```python
from build123d import *

# Parameters (mm, degrees)
EXTRUDE_1_DEPTH     = 2
SKETCH_2_R          = 1.05
CUT_EXTRUDE_1_DEPTH = 2
SKETCH_3_R          = 1.05
CUT_EXTRUDE_2_DEPTH = 2
FILLET_1_R          = 5
FILLET_2_R          = 1.5
SKETCH_5_R          = 1.6
CUT_EXTRUDE_4_DEPTH = 10
SKETCH_6_R          = 1.6
CUT_EXTRUDE_5_DEPTH = 10
CUT_EXTRUDE_6_DEPTH = 10
FILLET_3_R          = 2
FILLET_4_R          = 1.5
SKETCH_10_R         = 1.05
CUT_EXTRUDE_7_DEPTH = 10


with BuildPart() as part:
    # 草图1 → 凸台-拉伸1 (new body)
    with BuildSketch(Plane.XY):
        with BuildLine():
            Line((-53.112698372, 0), (-53.112698372, 20))
            Line((-53.112698372, 20), (-60.112698372, 20))
            Line((-60.112698372, 20), (-60.112698372, -60.112698372))
            Line((-60.112698372, -60.112698372), (10, -60.112698372))
            Line((10, -60.112698372), (10, -53.112698372))
            Line((10, -53.112698372), (0, -53.112698372))
            ThreePointArc((0, -53.112698372), (-37.556349186, -37.556349186), (-53.112698372, 0))
        make_face()
    extrude(amount=EXTRUDE_1_DEPTH)

    # 草图2 → 切除-拉伸1 (cut)
    with BuildSketch(Plane.XY.offset(2)):
        with Locations((5, -55.112698372)):
            Circle(SKETCH_2_R)
    extrude(amount=-CUT_EXTRUDE_1_DEPTH, mode=Mode.SUBTRACT)

    # 草图3 → 切除-拉伸2 (cut)
    with BuildSketch(Plane.XY.offset(2)):
        with Locations((-0.799997093, -55.106891824)):
            Circle(SKETCH_3_R)
        with Locations((-6.964981152, -54.670819999)):
            Circle(SKETCH_3_R)
        with Locations((-13.042376532, -53.547230893)):
            Circle(SKETCH_3_R)
        with Locations((-18.95575646, -51.750254288)):
            Circle(SKETCH_3_R)
        with Locations((-24.630756751, -49.30248821)):
            Circle(SKETCH_3_R)
        with Locations((-29.996010986, -46.234714737)):
            Circle(SKETCH_3_R)
        with Locations((-34.984047978, -42.5855129)):
            Circle(SKETCH_3_R)
        with Locations((-39.532140269, -38.400773529)):
            Circle(SKETCH_3_R)
        with Locations((-43.583092958, -33.733122151)):
            Circle(SKETCH_3_R)
        with Locations((-47.085962967, -28.641257189)):
            Circle(SKETCH_3_R)
        with Locations((-49.996699671, -23.1892118)):
            Circle(SKETCH_3_R)
        with Locations((-52.278698867, -17.445548618)):
            Circle(SKETCH_3_R)
        with Locations((-53.903263093, -11.48249754)):
            Circle(SKETCH_3_R)
        with Locations((-54.84996251, -5.375047393)):
            Circle(SKETCH_3_R)
        with Locations((-55.106891824, 0.799997093)):
            Circle(SKETCH_3_R)
    extrude(amount=-CUT_EXTRUDE_2_DEPTH, mode=Mode.SUBTRACT)

    # 圆角1
    fillet_1_edges = [part.edges().sort_by_distance(p)[0] for p in [
        (-60.112698372, -60.112698372, 1),
    ]]
    fillet(fillet_1_edges, radius=FILLET_1_R)

    # 圆角2
    fillet_2_edges = [part.edges().sort_by_distance(p)[0] for p in [
        (-60.112698372, 20, 1),
        (-53.112698372, 20, 1),
        (10, -53.112698372, 1),
        (10, -60.112698372, 1),
    ]]
    fillet(fillet_2_edges, radius=FILLET_2_R)

    # 草图5 → 切除-拉伸4 (cut)
    with BuildSketch(Plane.XY.offset(2)):
        with Locations((-57.199529996, -26.67257888)):
            Circle(SKETCH_5_R)
    extrude(amount=-CUT_EXTRUDE_4_DEPTH, mode=Mode.SUBTRACT)

    # 草图6 → 切除-拉伸5 (cut)
    with BuildSketch(Plane(origin=(0, 0, 0), x_dir=(-1, 0, 0), z_dir=(0, 0, -1))):
        with Locations((27, -57.112698372)):
            Circle(SKETCH_6_R)
        with Locations((47, -57.112698372)):
            Circle(SKETCH_6_R)
    extrude(amount=-CUT_EXTRUDE_5_DEPTH, mode=Mode.SUBTRACT)

    # 草图7 → 切除-拉伸6 (cut)
    with BuildSketch(Plane.XY.offset(2)):
        with BuildLine():
            Line((-55.112698372, -52.112698372), (-55.112698372, -26.407430403))
            ThreePointArc((-55.112698372, -26.407430403), (-45.375761756, -40.936562477), (-31.922226907, -52.112698372))
            Line((-31.922226907, -52.112698372), (-55.112698372, -52.112698372))
        make_face()
    extrude(amount=-CUT_EXTRUDE_6_DEPTH, mode=Mode.SUBTRACT)

    # 圆角3
    fillet_3_edges = [part.edges().sort_by_distance(p)[0] for p in [
        (-31.922226907, -52.112698372, 1),
        (-55.112698372, -26.407430403, 1),
    ]]
    fillet(fillet_3_edges, radius=FILLET_3_R)

    # 圆角4
    fillet_4_edges = [part.edges().sort_by_distance(p)[0] for p in [
        (-55.112698372, -52.112698372, 1),
    ]]
    fillet(fillet_4_edges, radius=FILLET_4_R)

    # 草图10 → 切除-拉伸7 (cut)
    with BuildSketch(Plane.XY.offset(2)):
        with Locations((-55.106891824, 0.799997093)):
            Circle(SKETCH_10_R)
        with Locations((-55.106891824, 6.599997093)):
            Circle(SKETCH_10_R)
        with Locations((-55.106891824, 12.399997093)):
            Circle(SKETCH_10_R)
    extrude(amount=-CUT_EXTRUDE_7_DEPTH, mode=Mode.SUBTRACT)


solid = part.part
```
Input: part model. Units: mm. Frame: model coordinates. A direction names the side the tool comes from. Give positions to 0.01 mm unless a question says otherwise; leave off trailing zeros. Order: outer loops, then holes, each group sorted by start corner. A loop starts at its lowest first (then second) coordinate and runs counter-clockwise, first axis right, second up. Notation, with made-up numbers: M -17.75,-26 L 34.25,-26 A13 cw 34.25,-12 Z; hole C 18.5,36.25 d11. An arc over 180 degrees is marked long. Return JSON: item names as keys, results as strings.
1) Mould query, pull axis Y, two halves, no side actions, for faces 1 (the face through (-58.687, -58.609, 1.014)), 2 (the face through (4, -53.113, 1)), 3 (the face through (-41, -35, 0)), 4 (the face through (-56.156, 0.846, 1.014)). Classes: released by +Y, released by -Y, zero draft, split by the parting line, or undercut.
Taken from the geometry:
{"face 1": "released by -Y", "face 2": "released by +Y", "face 3": "zero draft", "face 4": "undercut"}
2) Section query C-C on z = 0.3. Count the separate pieces of the cut face and the enclosed holes in it, and give its area (3 significant figures).
Taken from the geometry:
{"separate pieces": "1", "enclosed holes": "22", "area": "1,290 mm2"}
3) Section query A-A on x = 5. Output: boundary loops of the cut face in (y, z), and give its area (3 significant figures).
Taken from the geometry:
{"outline": "M -60.11,0 L -56.16,0 L -56.16,2 L -60.11,2 Z; M -54.06,0 L -53.11,0 L -53.11,2 L -54.06,2 Z", "area": "9.80 mm2"}
4) Access query for faces 5 (the face through (-37.14, -37.97, 0.99)), 6 (the face through (-53.641, -32.163, 0.986)). Directions: +Z, -Z, +X, -X, +Y, -Y. A direction counts if a zero-diameter tool reaches every point of the face in a straight line with its end or side. Return the directions, or none.
Taken from the geometry:
{"face 5": "+Z, -Z, +X, +Y", "face 6": "+Z, -Z"}
5) Section query D-D on x = -27. Output: boundary loops of the cut face in (y, z), and give its area (3 significant figures).
Taken from the geometry:
{"outline": "M -60.11,0 L -58.71,0 L -58.71,2 L -60.11,2 Z; M -55.51,0 L -45.74,0 L -45.74,2 L -55.51,2 Z", "area": "22.3 mm2"}
6) Section query B-B on x = -47. Output: boundary loops of the cut face in (y, z), and give its area (3 significant figures).
Taken from the geometry:
{"outline": "M -60.11,0 L -58.71,0 L -58.71,2 L -60.11,2 Z; M -55.51,0 L -52.11,0 L -52.11,2 L -55.51,2 Z; M -39.06,0 L -29.69,0 L -29.69,2 L -39.06,2 Z; M -27.59,0 L -24.74,0 L -24.74,2 L -27.59,2 Z", "area": "34.1 mm2"}
7) Line query: L1, parallel to X at y = -49, z = 0.45; L2, parallel to Y at x = -56, z = 1.8; L3, parallel to X at y = -42.5, z = 1.45. Output: solid intervals per line, ascending. Write a range as [from, to].
Taken from the geometry:
{"L1": "x = [-60.11, -55.11], [-36.7, -25.64], [-23.63, -20.49]", "L2": "y = [-60.03, -27.73], [-25.61, 0.25], [1.35, 6.05], [7.15, 11.85], [12.95, 20]", "L3": "x = [-60.11, -55.11], [-43.91, -36.03], [-33.94, -31.85]"}
